Study the drawing (mm; zero at the part's minimum x, y, z) and answer. Coordinates: 2 decimals unless noted, no trailing zeros. Loops run counter-clockwise (first coordinate to the right, second up) from the corner with the lowest first, then second, coordinate; pieces in that order, holes last. Notation, with made-up numbers: (40.25, -18) -> (98.25, -18) arc R17 cw to (98.25, 11) -> close; hole circle Ø1 at (89.5, 53). An arc over 180 degrees is marked (long way). Answer as CSV lines item,"result".
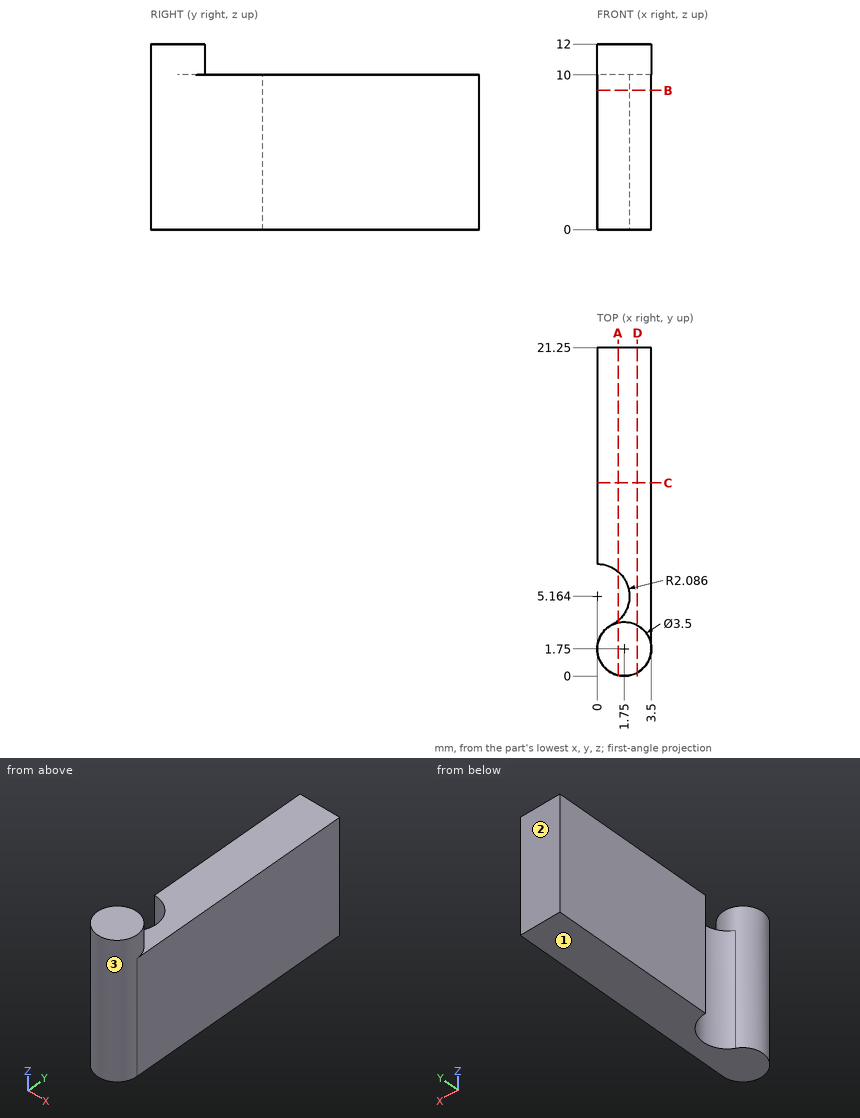
Q1. Given pin 1 Ø1 at (x, y) = (1.5, 15) entering from +Z, flat-ended and moving along its own axis, determine where the tip first touches the part or whether it passes through.
Results:
pin 1,"stops at z = 10"
Q2. A cutting plane is placed at D-D, the plane x = 2.6. Write down the section's boundary in (y, z).
Results:
outline,"(0.22, 0) -> (21.25, 0) -> (21.25, 10) -> (3.28, 10) -> (3.28, 12) -> (0.22, 12) -> close"
Q3. A cutting plane is placed at A-A, the plane x = 1.35. Write down the section's boundary in (y, z), and give its area (3 significant figures).
Results:
outline,"(0.05, 0) -> (3.57, 0) -> (3.57, 10) -> (3.45, 10) -> (3.45, 12) -> (0.05, 12) -> close; (6.75, 0) -> (21.25, 0) -> (21.25, 10) -> (6.75, 10) -> close"
area,"187 mm²"
Q4. For a pull along Y with two mould halves and no side action, classify the marked faces 1, 2 and 3 as pulls with the +Y half, pulls with the -Y half, needs draft (parallel to the pull), parting line crosses it, or undercut.
Results:
face 1,"needs draft"
face 2,"pulls with the +Y half"
face 3,"undercut"
Q5. Find the intervals of material crossed by probe 1 along Z at (x, y) = (3.15, 20); probe 2 along Y at (x, z) = (0.95, 5); probe 3 along Y at (x, z) = (0.9, 10.25), in increasing order. Write a range as [from, to].
Results:
probe 1,"z = [0, 10]"
probe 2,"y = [0.19, 3.31], [7.02, 21.25]"
probe 3,"y = [0.22, 3.28]"
Q6. A cutting plane is placed at C-C, the plane y = 12.5. Write down the section's boundary in (x, z).
Results:
outline,"(0, 0) -> (3.5, 0) -> (3.5, 10) -> (0, 10) -> close"
Q7. A cutting plane is placed at B-B, the plane z = 9. Write down the section's boundary in (x, y).
Results:
outline,"(0, 7.25) arc R2.09 cw to (0.95, 3.31) arc R1.75 ccw (long way) to (3.5, 1.75) -> (3.5, 21.25) -> (0, 21.25) -> close"
